The figure shows three views and two pictorial views of one solid part (mm, origin at its lowest corner). Answer the questions. Round coordinates to 2 decimals unless told otherwise and drop trailing zeros.
Item 1: Each of these flat-tipped pins is pushed along its axis until it touches: pin 1 (1 mm diameter, centred on x = 2, y = 2, fed in from -Z); pin 2 (3 mm diameter, centred on y = 2, z = 1, fed in from -X); pin 3 (1 mm diameter, centred on x = 5, y = 2, fed in from -Z). Where does it stop, or does it pass through?
Item 2: Find the intervals of material crossed by probe 1 along Z at (x, y) = (2, 2.65); probe 2 along Z at (x, y) = (4.75, 2.5) (1 decimal); probe 3 along X at (y, z) = (2.25, 1.75) (1 decimal), in increasing order.
Item 3: For a pull along Z with two mould halves and no side action, classify the marked faces 1, 2 and 3 as +Z half, -Z half, draft (parallel to the pull), parting line (faces both ways), or undercut.
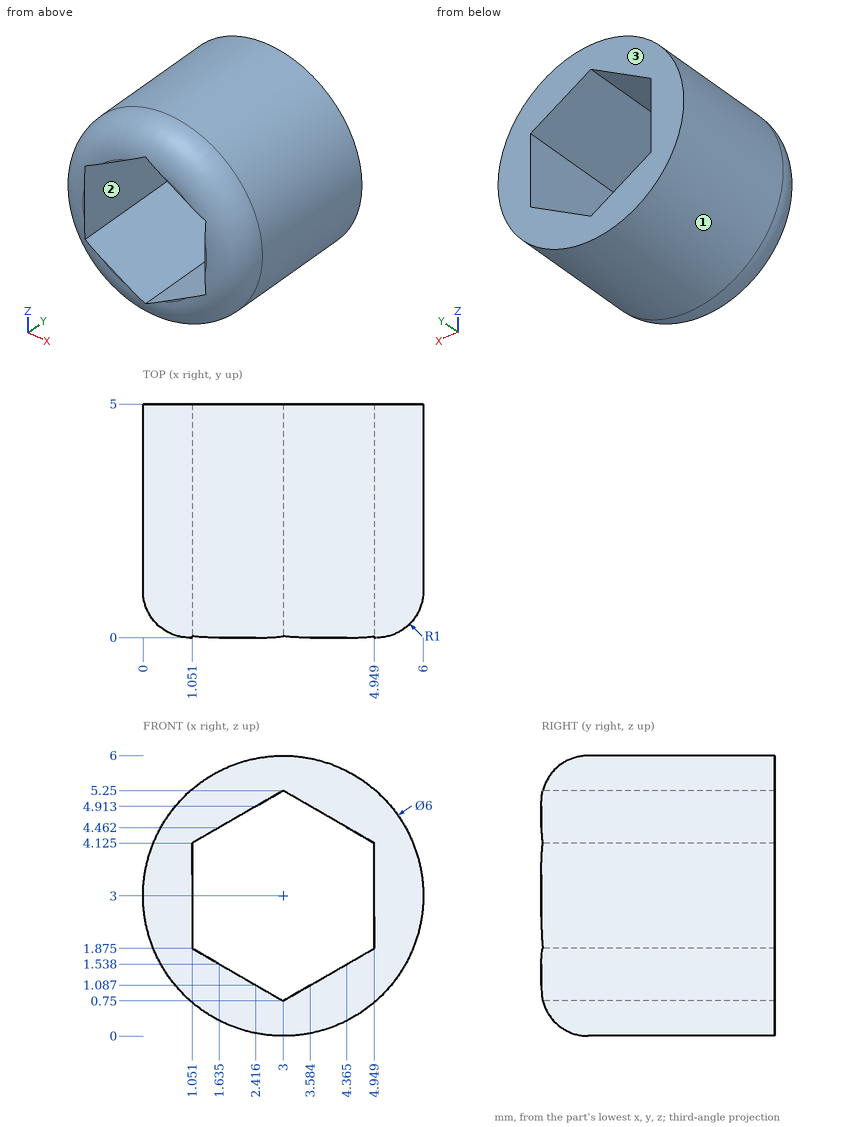
Check values:
1. pin 1: stops at z = 0.04
1. pin 2: stops at x = 0.04
1. pin 3: stops at z = 0.4
2. probe 1: z = 0.17 to 1.33, 4.67 to 5.83
2. probe 2: z = 0.6 to 1.8, 4.2 to 5.4
2. probe 3: x = 0.3 to 1.3, 4.7 to 5.7
3. face 1: parting line
3. face 2: undercut
3. face 3: draft
